from build123d import *

# Parameters (mm, degrees)
SKETCH1_W              = 130
SKETCH1_H              = 100
BASE_FLANGE1_DEPTH     = 3
SKETCHED_START         = -50
SKETCHED_BEND1_DEPTH   = 100
SKETCHED_BEND1_2_DEPTH = 100


# Read off the part's stored shape, not the designer's step: Sketched Bend1
# Sheet-metal steps are written as plain solids
with BuildPart() as part:
    # Sketch1 → Base-Flange1 (new body)
    with BuildSketch(Plane(origin=(0, 0, 0), x_dir=(1, 0, 0), z_dir=(0, 1, 0))):
        Rectangle(SKETCH1_W, SKETCH1_H)
    extrude(amount=-BASE_FLANGE1_DEPTH)

    # Sketched Bend1 outline → Sketched Bend1 (cut)
    with BuildSketch(Plane.XY.offset(SKETCHED_START)):
        with BuildLine():
            Line((-65, -3), (-30, -3))
            ThreePointArc((-30, -3), (-32.738612788, -2.183300133), (-34.582575695, 0))
            Line((-34.582575695, 0), (-65, 0))
            Line((-65, 0), (-65, -3))
        make_face()
        with BuildLine():
            ThreePointArc((34.582575695, 0), (32.738612788, -2.183300133), (30, -3))
            Line((30, -3), (65, -3))
            Line((65, -3), (65, 0))
            Line((65, 0), (34.582575695, 0))
        make_face()
    extrude(amount=SKETCHED_BEND1_DEPTH, mode=Mode.SUBTRACT)

    # Sketched Bend1 2 outline → Sketched Bend1 2 (add)
    with BuildSketch(Plane.XY.offset(SKETCHED_START)):
        with BuildLine():
            ThreePointArc((-35, 2), (-34.894531565, 0.978451782), (-34.582575695, 0))
            Line((-34.582575695, 0), (-30, 0))
            ThreePointArc((-30, 0), (-31.414213562, 0.585786438), (-32, 2))
            Line((-32, 2), (-32, 31.502212856))
            Line((-32, 31.502212856), (-35, 31.502212856))
            Line((-35, 31.502212856), (-35, 2))
        make_face()
        with BuildLine():
            Line((30, 0), (34.582575695, 0))
            ThreePointArc((34.582575695, 0), (34.894531565, 0.978451782), (35, 2))
            Line((35, 2), (35, 31.502212856))
            Line((35, 31.502212856), (32, 31.502212856))
            Line((32, 31.502212856), (32, 2))
            ThreePointArc((32, 2), (31.414213562, 0.585786438), (30, 0))
        make_face()
    extrude(amount=SKETCHED_BEND1_2_DEPTH)


solid = part.part
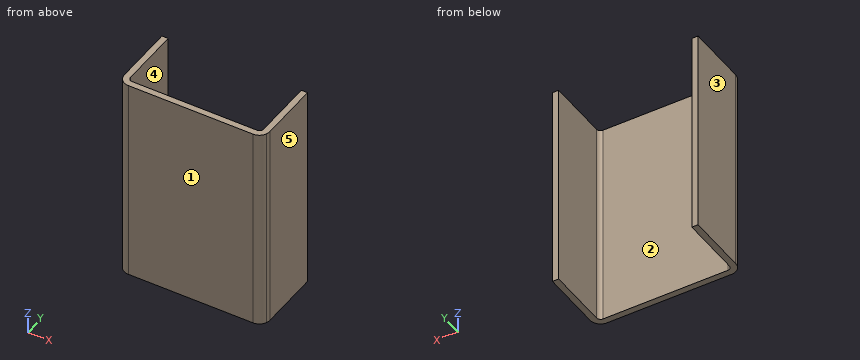
Design review of the part built by this model. Coordinates are the model's own, in mm. Face numbers are marked on the shaded views. A direction names the side the tool comes from. Coordinates: 2 decimals unless noted, no trailing zeros. Order: outer loops, then holes, each group sorted by start corner. A loop starts at its lowest first (then second) coordinate and runs counter-clockwise, first axis right, second up. Notation, with made-up numbers: (82.5, 30.25) - (103.5, 30.25) arc R17 ccw to (103.5, 48.25) - close; hole circle Ø3 at (20.5, 28). An arc over 180 degrees is marked (long way). Put each result on its own line as item: value.
1) Wall thickness on L1, parallel to X at y = 6.5, z = 11; L2, parallel to Y at x = -12.5, z = -37: over which ranges is each line inside the solid? List them lowest first. Write a range as from..to.
Response values:
L1: x = -35..-32, 32..35
L2: y = -3..0
2) Take a section at A-A, the plane y = 9. Give the boundary of the cut face in (x, z), and give its area (3 significant figures).
Response values:
outline: (-35, -50) - (-32, -50) - (-32, 50) - (-35, 50) - close; (32, -50) - (35, -50) - (35, 50) - (32, 50) - close
area: 600 mm²
3) Tool access review of the marked faces 4 and 5: name each direction out of +Z, -Z, +X, -X, +Y, -Y from which nothing blocks a thin tool from reaching the whole face with its end or side.
Response values:
face 4: +Z, -Z, +Y
face 5: +Z, -Z, +X, +Y, -Y
4) Take a section at B-B, the plane z = -3.5. Give the boundary of the cut face in (x, y).
Response values:
outline: (-35, 2) arc R5 ccw to (-30, -3) - (30, -3) arc R5 ccw to (35, 2) - (35, 31.5) - (32, 31.5) - (32, 2) arc R2 cw to (30, 0) - (-30, 0) arc R2 cw to (-32, 2) - (-32, 31.5) - (-35, 31.5) - close
5) Take a section at C-C, the plane x = 20.5. Give the boundary of the cut face in (y, z), and give its area (3 significant figures).
Response values:
outline: (-3, -50) - (0, -50) - (0, 50) - (-3, 50) - close
area: 300 mm²
6) Insertion check: P1, Ø1, axis at x = 19.5, z = -30, coming from the +Y side. The pin has a flat end and moves straight along its axis. Give the tip position at first contact, or say it passes through.
Response values:
P1: stops at y = 0
7) The part is to be moulded in two halves that separate along X. For the marked faces 1, 2 and 3, say which applies: released by +X, released by -X, zero draft, split by the parting line, or undercut.
Response values:
face 1: zero draft
face 2: undercut
face 3: released by -X
